Geometry check sheet. Reference: drawing and pictorial views, mm from the part's lowest x, y, z. A direction names the side the tool comes from. Round coordinates to 2 decimals unless told otherwise and drop trailing zeros. Write each loop counter-clockwise with the first axis right and the second up, starting at its lowest first coordinate (ties: lowest second). Pieces come first, ordered by that corner, then holes. Notation, with made-up numbers: M 17.25,-6.75 L 64.25,-6.75 A30 cw 64.25,20.25 Z; hole C 60,84 d8. An arc over 180 degrees is marked long. One line per question, with ' | ' between items.
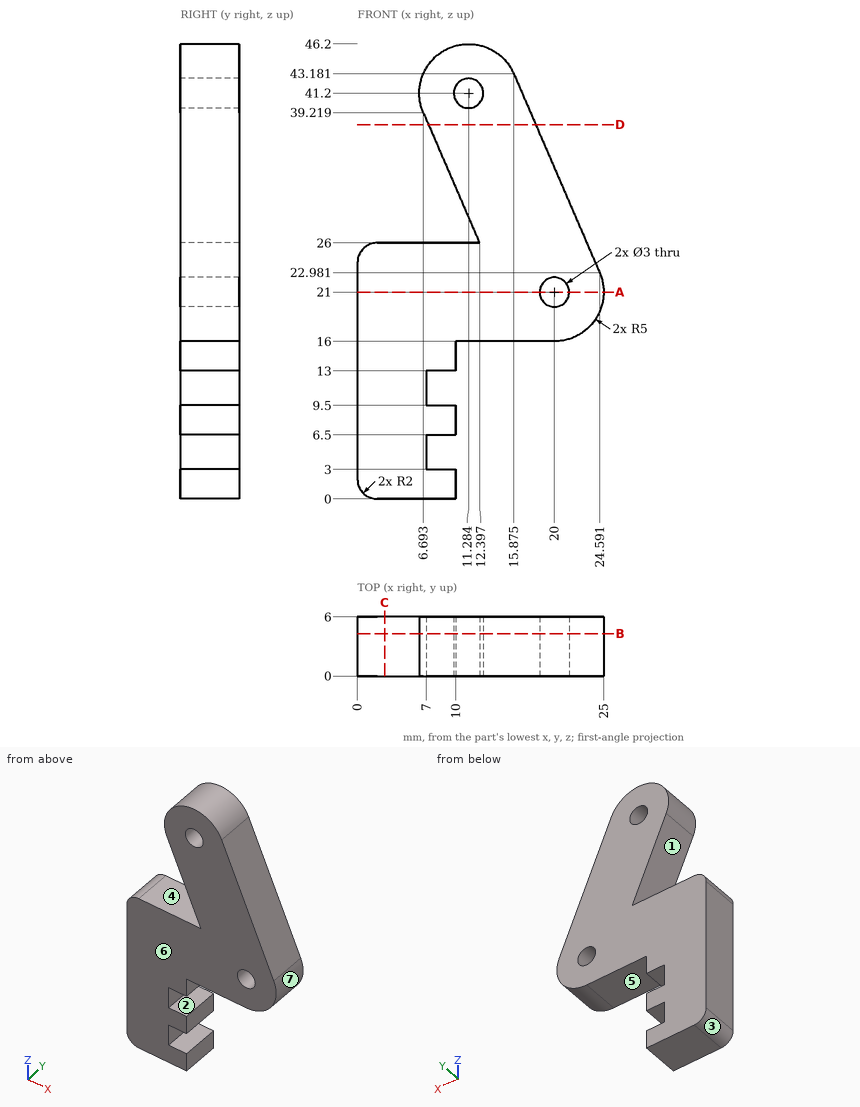
1. Section check D-D, the plane z = 38. Record the cut outline in (x, y).
Results:
outline: M 7.22,0 L 18.11,0 L 18.11,6 L 7.22,6 Z
2. Tool access check on the marked faces 1, 2 and 3. Record the directions out of +Z, -Z, +X, -X, +Y, -Y that give a thin tool (end or side, any length) a straight path to the whole face; none if there is none.
Results:
face 1: -X, +Y, -Y | face 2: +X, +Y, -Y | face 3: -Z, -X, +Y, -Y
3. Thickness scan on line 1 (X direction, y = 2.65, z = 21); line 2 (Z direction, x = 11.5, y = 3.8) (1 decimal); line 3 (Z direction, x = 9.25, y = 4.4) (1 decimal). Record the ranges inside material, lowest first.
Results:
line 1: x = 0 to 18.5, 21.5 to 25 | line 2: z = 16 to 26, 28.1 to 39.7, 42.7 to 46.2 | line 3: z = 0 to 3, 6.5 to 9.5, 13 to 26, 33.3 to 45.8
4. Section check C-C, the plane x = 2.75. Record the cut outline in (y, z).
Results:
outline: M 0,0 L 6,0 L 6,26 L 0,26 Z
5. Section check B-B, the plane y = 4.3. Record the cut outline in (x, z) (1 decimal).
Results:
outline: M 0,2 A2 ccw 2,0 L 10,0 L 10,3 L 7,3 L 7,6.5 L 10,6.5 L 10,9.5 L 7,9.5 L 7,13 L 10,13 L 10,16 L 20,16 A5 ccw 24.6,23 L 15.9,43.2 A5 ccw 6.7,39.2 L 12.4,26 L 2,26 A2 ccw 0,24 Z; hole C 11.3,41.2 d3; hole C 20,21 d3
6. Go/stop test with flat-tipped pins: P1, Ø1.8, axis at y = 4, z = 5.5, coming from the +X side; P2, Ø0.9, axis at x = 9, y = 2.5, coming from the +Z side; P3, Ø3, axis at y = 4.5, z = 36.5, coming from the -X side. Record where each tip stops, or that it passes through.
Results:
P1: stops at x = 7 | P2: stops at z = 45.85 | P3: stops at x = 7.22
7. Mould release check, pull along Z, two halves, no side actions. Record for the marked faces 4, 5, 6 and 7: pulls with the +Z half, pulls with the -Z half, needs draft (parallel to the pull), parting line crosses it, or undercut.
Results:
face 4: undercut | face 5: pulls with the -Z half | face 6: needs draft | face 7: parting line crosses it
8. Section check A-A, the plane z = 21. Record the cut outline in (x, y), then the cut area to 3 significant figures.
Results:
outline: M 0,0 L 18.5,0 L 18.5,6 L 0,6 Z; M 21.5,0 L 25,0 L 25,6 L 21.5,6 Z | area: 132 mm2
